from build123d import *

# Parameters (mm, degrees)
SKETCH_1_W          = 25
SKETCH_1_H          = 20
EXTRUDE_1_DEPTH     = 38.8
SKETCH_3_W          = 4.4
SKETCH_3_H          = 10
EXTRUDE_2_DEPTH     = 38.8
SKETCH_5_W          = 15
SKETCH_5_H          = 38.8
CUT_EXTRUDE_2_DEPTH = 2.2


with BuildPart() as part:
    # 草圖1 → 填料-伸長1 (new body)
    with BuildSketch(Plane(origin=(0, 0, 0), x_dir=(1, 0, 0), z_dir=(0, 1, 0))):
        Rectangle(SKETCH_1_W, SKETCH_1_H)
    extrude(amount=EXTRUDE_1_DEPTH)

    # 草圖3 → 填料-伸長2 (add)
    with BuildSketch(Plane(origin=(0, 38.8, 0), x_dir=(1, 0, 0), z_dir=(0, 1, 0))):
        with Locations((0, -15)):
            Rectangle(SKETCH_3_W, SKETCH_3_H)
    extrude(amount=-EXTRUDE_2_DEPTH)

    # 草圖5 → 除料-伸長2 (cut)
    with BuildSketch(Plane(origin=(2.2, 0, 0), x_dir=(0, 0, -1), z_dir=(1, 0, 0))):
        with Locations((-12.5, 19.4)):
            Rectangle(SKETCH_5_W, SKETCH_5_H)
    extrude(amount=-CUT_EXTRUDE_2_DEPTH, mode=Mode.SUBTRACT)


solid = part.part
Verification items for the finished model (mm, model axes). A direction names the side the tool comes from. Give positions to 0.01 mm unless a question says otherwise; leave off trailing zeros. Write each loop counter-clockwise with the first axis right and the second up, starting at its lowest first coordinate (ties: lowest second). Pieces come first, ordered by that corner, then holes. Notation, with made-up numbers: (33, -15.5) - (56, -15.5) arc R22 cw to (56, 19.5) - close; hole circle Ø9 at (31, -34.75). An arc over 180 degrees is marked (long way). Answer as CSV lines item,"result". Start each with the question number.
1. Thickness scan on line 1 (X direction, y = 20.5, z = 9.5); line 2 (Z direction, x = -4, y = 14.5); line 3 (Z direction, x = 1, y = 10). Record the ranges inside material, lowest first.
2. Sectioned sample at B-B (y = 6). Record the boundary of the cut face in (x, z).
3. Sectioned sample at C-C (z = 14). Record the boundary of the cut face in (x, y).
4. Draft check along X on faces 1 (the face through (12.5, 19, 0)), 2 (the face through (0, 19, -10)), 3 (the face through (0, 20, 13)), 4 (the face through (-2.2, 20, 15)). Enter one of: pulls with the +X half, pulls with the -X half, needs draft (parallel to the pull), parting line crosses it, or undercut.
5. Depth check by flat-ended pin: pin 1 (5 mm diameter, centred on x = -7.5, y = 21.5, fed in from +Z); pin 2 (4.5 mm diameter, centred on y = 18.5, z = 14.5, fed in from +X); pin 3 (10 mm diameter, centred on x = -7, z = -1, fed in from -Y). Enter the tip coordinate at first touch or a pass-through.
6. Set-up check for faces 5 (the face through (7, 19, 10)), 6 (the face through (0, 38.8, 1)), 7 (the face through (0, 0, 1)), 8 (the face through (-7, 19, 10)), 9 (the face through (2.2, 20, 8)): record each of +Z, -Z, +X, -X, +Y, -Y from which the full face is reachable in a straight line by a thin tool's end or side.
7. Sectioned sample at D-D (x = 3.75). Record the boundary of the cut face in (y, z), then the cut area to 3 significant figures.
8. Sectioned sample at A-A (z = 9). Record the boundary of the cut face in (x, y).
Derived:
1,line 1,"-12.5 to 0, 2.2 to 12.5"
1,line 2,"-10 to 10"
1,line 3,"-10 to 5"
2,outline,"(-12.5, -10) - (12.5, -10) - (12.5, 10) - (2.2, 10) - (2.2, 5) - (0, 5) - (0, 20) - (-2.2, 20) - (-2.2, 10) - (-12.5, 10) - close"
3,outline,"(-2.2, 0) - (0, 0) - (0, 38.8) - (-2.2, 38.8) - close"
4,face 1,"pulls with the +X half"
4,face 2,"needs draft"
4,face 3,"undercut"
4,face 4,"pulls with the -X half"
5,pin 1,"z = 10"
5,pin 2,"x = 0"
5,pin 3,"y = 0"
6,face 5,"+Z, +X, +Y, -Y"
6,face 6,"+Z, -Z, +X, -X, +Y"
6,face 7,"+Z, -Z, +X, -X, -Y"
6,face 8,"+Z, -X, +Y, -Y"
6,face 9,"+Z, +Y, -Y"
7,outline,"(0, -10) - (38.8, -10) - (38.8, 10) - (0, 10) - close"
7,area,"776 mm²"
8,outline,"(-12.5, 0) - (0, 0) - (0, 38.8) - (-12.5, 38.8) - close; (2.2, 0) - (12.5, 0) - (12.5, 38.8) - (2.2, 38.8) - close"
